Drawing for the job (mm, zero at the part's lowest x, y, z). A direction names the side the tool comes from. Coordinates: 2 decimals unless noted, no trailing zeros. Order: outer loops, then holes, each group sorted by start corner. A loop starts at its lowest first (then second) coordinate and runs counter-clockwise, first axis right, second up.
1) Mould opens along X. For the marked faces 4, 5 and 6 say: +X half, -X half, draft (parallel to the pull), parting line (faces both ways), or undercut.
2) Cut at C-C (x = 16.5). List the corners of the cut face in (y, z).
3) Wall check: L1, parallel to X at y = 51, z = 4.5; L2, parallel to Z at x = 2.7, y = 17. Give the ranges that are in metal, low to high.
4) Pin check, flat tips, straight feed: pin 1 Ø3.5 at (y, z) = (40, 6) entering from +X; pin 2 Ø6 at (x, y) = (11, 33.5) entering from +Z; pin 3 Ø3.5 at (x, z) = (42, 4.5) entering from -Y. Stop position of each tip, or through.
5) Cut at B-B (z = 5). List the corners of the cut face in (x, y), and give its area (3 significant figures).
6) Cut at A-A (y = 53). List the corners of the cut face in (x, z).
7) Tool access for the marked faces 1, 2 and 3: list every direction of +Z, -Z, +X, -X, +Y, -Y with a clear straight run to the whole face (end or side of a thin tool).
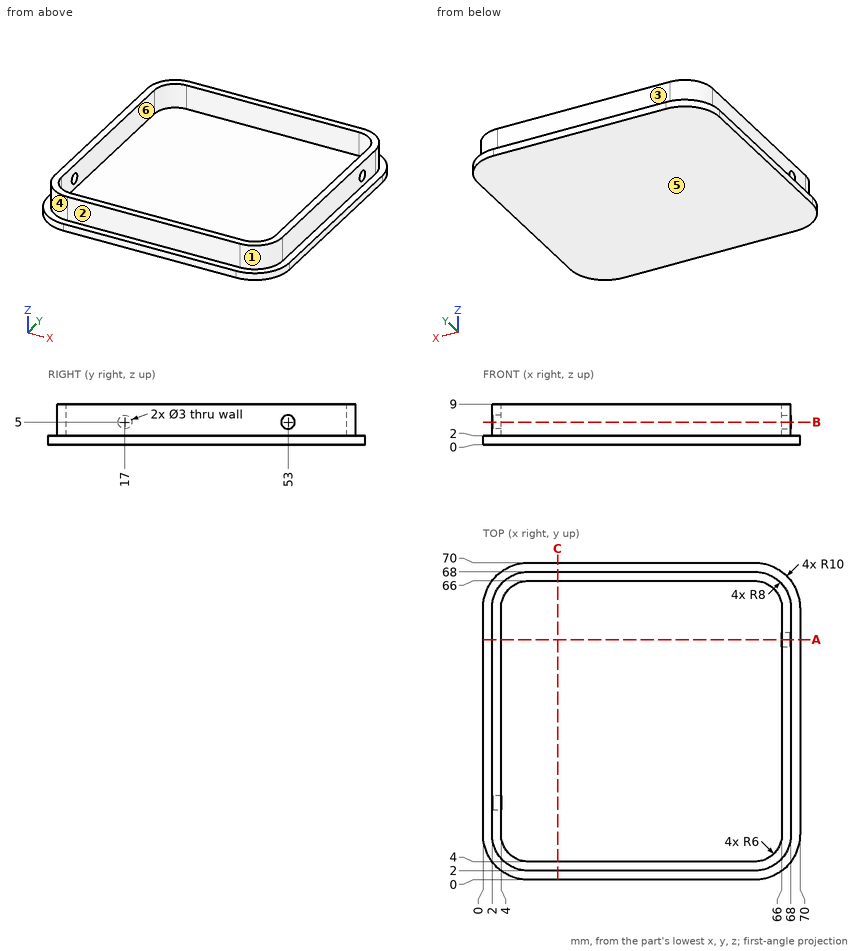
Geometry check:
1. face 4: -X half
1. face 5: draft
1. face 6: undercut
2. outline: (0, 0) - (70, 0) - (70, 2) - (68, 2) - (68, 9) - (66, 9) - (66, 2) - (4, 2) - (4, 9) - (2, 9) - (2, 2) - (0, 2) - close
3. L1: x = 2 to 4, 66 to 68
3. L2: z = 0 to 3.5, 6.5 to 9
4. pin 1: stops at x = 68
4. pin 2: stops at z = 2
4. pin 3: stops at y = 2
5. outline: (2, 10) arc R8 ccw to (10, 2) - (60, 2) arc R8 ccw to (68, 10) - (68, 51.5) - (66, 51.5) - (66, 10) arc R6 cw to (60, 4) - (10, 4) arc R6 cw to (4, 10) - (4, 15.5) - (2, 15.5) - close; (2, 18.5) - (4, 18.5) - (4, 60) arc R6 cw to (10, 66) - (60, 66) arc R6 cw to (66, 60) - (66, 54.5) - (68, 54.5) - (68, 60) arc R8 ccw to (60, 68) - (10, 68) arc R8 ccw to (2, 60) - close
5. area: 476 mm2
6. outline: (0, 0) - (70, 0) - (70, 2) - (68, 2) - (68, 3.5) - (66, 3.5) - (66, 2) - (4, 2) - (4, 9) - (2, 9) - (2, 2) - (0, 2) - close; (66, 6.5) - (68, 6.5) - (68, 9) - (66, 9) - close
7. face 1: +Z, +X, -Y
7. face 2: +Z, +X, -X, -Y
7. face 3: +Z, +X, -X, +Y
